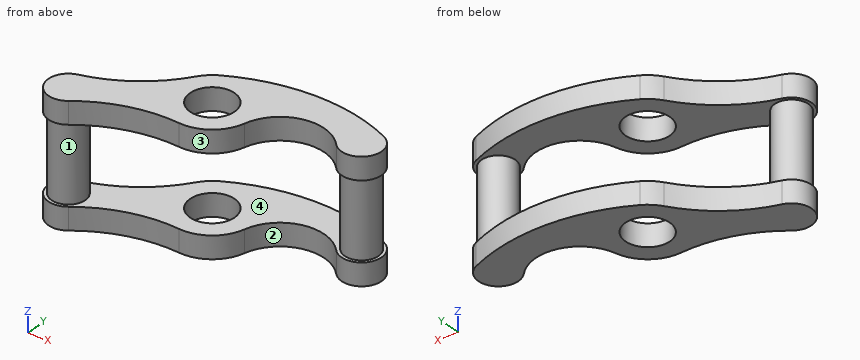
```python
from build123d import *

# Parameters (mm, degrees)
CROQUIS1_R              = 2.5
SALIENTE_EXTRUIR1_DEPTH = 2.5
CROQUIS2_R              = 1.9
SALIENTE_EXTRUIR2_DEPTH = 8.6
CROQUIS3_R              = 2.5
SALIENTE_EXTRUIR3_DEPTH = 2.5


with BuildPart() as part:
    # Croquis1 → Saliente-Extruir1 (new body)
    with BuildSketch(Plane.XY):
        with BuildLine():
            ThreePointArc((-0.171650138, -4.496725056), (2.753921849, -3.558920405), (4.395901196, -0.962316307))
            ThreePointArc((4.395901196, -0.962316307), (7.9188241, 2.779530342), (12.880073197, 1.43848242))
            ThreePointArc((12.880073197, 1.43848242), (16.361169276, 1.735662654), (15.354744139, 5.081324688))
            ThreePointArc((15.354744139, 5.081324688), (6.413547413, 6.535486918), (-2.252037616, 3.895937188))
            ThreePointArc((-2.252037616, 3.895937188), (-3.106745208, 3.25547757), (-3.786445073, 2.431631903))
            ThreePointArc((-3.786445073, 2.431631903), (-7.399355323, -1.45649364), (-12.140164606, -3.842990664))
            ThreePointArc((-12.140164606, -3.842990664), (-13.494815904, -7.040773515), (-10.097019643, -7.75901851))
            ThreePointArc((-10.097019643, -7.75901851), (-5.427542776, -5.235801021), (-0.171650138, -4.496725056))
        make_face()
        Circle(CROQUIS1_R, mode=Mode.SUBTRACT)
    extrude(amount=SALIENTE_EXTRUIR1_DEPTH)

    # Croquis2 → Saliente-Extruir2 (add)
    with BuildSketch(Plane.XY.offset(2.5)):
        with Locations(Location((-11.5, -6, 0), (0, 0, 180))):
            Circle(CROQUIS2_R)
        with Locations(Location((14.5, 3, 0), (0, 0, 180))):
            Circle(CROQUIS2_R)
    extrude(amount=SALIENTE_EXTRUIR2_DEPTH)

    # Croquis3 → Saliente-Extruir3 (add)
    with BuildSketch(Plane.XY.offset(11.1)):
        with BuildLine():
            ThreePointArc((12.880073197, 1.43848242), (16.361169276, 1.735662654), (15.354744139, 5.081324688))
            ThreePointArc((15.354744139, 5.081324688), (6.413547413, 6.535486918), (-2.252037616, 3.895937188))
            ThreePointArc((-2.252037616, 3.895937188), (-3.106745208, 3.25547757), (-3.786445073, 2.431631903))
            ThreePointArc((-3.786445073, 2.431631903), (-7.399355323, -1.45649364), (-12.140164606, -3.842990664))
            ThreePointArc((-12.140164606, -3.842990664), (-13.494815904, -7.040773515), (-10.097019643, -7.75901851))
            ThreePointArc((-10.097019643, -7.75901851), (-5.427542776, -5.235801021), (-0.171650138, -4.496725056))
            ThreePointArc((-0.171650138, -4.496725056), (2.753921849, -3.558920405), (4.395901196, -0.962316307))
            ThreePointArc((4.395901196, -0.962316307), (7.9188241, 2.779530342), (12.880073197, 1.43848242))
        make_face()
        Circle(CROQUIS3_R, mode=Mode.SUBTRACT)
    extrude(amount=SALIENTE_EXTRUIR3_DEPTH)


solid = part.part
```
For this review, take the finished solid that the model builds, in its own axes (mm). Face numbers are marked on the shaded views. A direction names the side the tool comes from. Round coordinates to 2 decimals unless told otherwise and drop trailing zeros. Write each loop counter-clockwise with the first axis right and the second up, starting at its lowest first coordinate (ties: lowest second). Pieces come first, ordered by that corner, then holes. Notation, with made-up numbers: M 84,2.5 L 116,2.5 A31 cw 116,32.5 Z; hole C 36,63.25 d1. An arc over 180 degrees is marked long. One line per item, written item: value. Start each with the question number.
(1) Wall thickness on line 1 (Z direction, x = 6.5, y = 3); line 2 (X direction, y = -1.25, z = 1.5); line 3 (Y direction, x = 0, z = 11.95): over which ranges is each line inside the solid? List them lowest first.
(2) We need section D-D (z = 7). Give the boundary of the cut face in (x, y), and give its area (3 significant figures).
(3) The part is to be moulded in two halves that separate along Z. For the marked faces 3 and 4, say which applies: released by +Z, released by -Z, zero draft, split by the parting line, or undercut.
(4) Machinability: for the marked faces 1 and 2, which of the approach directions +Z, -Z, +X, -X, +Y, -Y give a long, thin tool a straight path to every point of the face, cutting with its end or side? Answer none if there is none.
(5) We need section A-A (x = 12). Give the boundary of the cut face in (y, z).
(6) We need section B-B (x = 1). Give the boundary of the cut face in (y, z), and give its area (3 significant figures).
(7) Insertion check: pin 1 (3 mm diameter, centred on y = 5, z = 12, fed in from -X); pin 2 (1.5 mm diameter, centred on y = 1.5, z = 11, fed in from -X); pin 3 (2 mm diameter, centred on x = -1, y = 1, fed in from +Z); pin 4 (3 mm diameter, centred on y = 3, z = 7.5, fed in from +X). Each pin has a flat end and moves straight along its axis. Give the tip position at first contact, or say it passes through.
(8) We need section C-C (y = 0). Give the boundary of the cut face in (x, z).
Result:
1. line 1: 0 to 2.5, 11.1 to 13.6
1. line 2: -7.13 to -2.17, 2.17 to 4.32
1. line 3: -4.5 to -2.5, 2.5 to 5.02
2. outline: C -11.5,-6 d3.8; C 14.5,3 d3.8
2. area: 22.7 mm²
3. face 3: zero draft
3. face 4: undercut
4. face 1: none
4. face 2: +Z, -Z, -Y
5. outline: M 2.16,0 L 6.13,0 L 6.13,2.5 L 2.16,2.5 Z; M 2.16,11.1 L 6.13,11.1 L 6.13,13.6 L 2.16,13.6 Z
6. outline: M -4.39,0 L -2.29,0 L -2.29,2.5 L -4.39,2.5 Z; M -4.39,11.1 L -2.29,11.1 L -2.29,13.6 L -4.39,13.6 Z; M 2.29,0 L 5.4,0 L 5.4,2.5 L 2.29,2.5 Z; M 2.29,11.1 L 5.4,11.1 L 5.4,13.6 L 2.29,13.6 Z
6. area: 26.0 mm²
7. pin 1: x = -2.83
7. pin 2: x = -5.03
7. pin 3: through
7. pin 4: x = 16.4
8. outline: M -5.73,0 L -2.5,0 L -2.5,2.5 L -5.73,2.5 Z; M -5.73,11.1 L -2.5,11.1 L -2.5,13.6 L -5.73,13.6 Z; M 2.5,0 L 4.71,0 L 4.71,2.5 L 2.5,2.5 Z; M 2.5,11.1 L 4.71,11.1 L 4.71,13.6 L 2.5,13.6 Z
